Here's how the part is built. I have some questions about the finished solid (model axes, mm). A direction names the side the tool comes from. Round coordinates to 2 decimals unless told otherwise and drop trailing zeros. Write each loop counter-clockwise with the first axis right and the second up, starting at its lowest first coordinate (ties: lowest second). Pieces come first, ordered by that corner, then holes. Notation, with made-up numbers: (34, 23.5) - (48, 23.5) arc R25 ccw to (48, 41.5) - close; hole circle Ø2 at (29.25, 19). An arc over 180 degrees is marked (long way). Return JSON: item names as keys, results as strings. Group by question number.
```python
from build123d import *

# Parameters (mm, degrees)
SKETCH1_W           = 12.7
SKETCH1_H           = 12.7
BOSS_EXTRUDE1_DEPTH = 1.7
CHAMFER3_SIZE       = 1.41
SKETCH2_R           = 1.2
CUT_EXTRUDE2_DEPTH  = 2.7
SKETCH3_R           = 3.15
SKETCH3_R_2         = 2.2
BOSS_EXTRUDE2_DEPTH = 7.8
SKETCH4_R           = 0.64
BOSS_EXTRUDE3_DEPTH = 5


with BuildPart() as part:
    # Sketch1 → Boss-Extrude1 (new body)
    with BuildSketch(Plane(origin=(0, 0, 0), x_dir=(0, 1, 0), z_dir=(0, 0, 1))):
        Rectangle(SKETCH1_W, SKETCH1_H)
    extrude(amount=BOSS_EXTRUDE1_DEPTH)

    # Chamfer3
    chamfer3_edges = [part.edges().sort_by_distance(p)[0] for p in [
        (6.35, 6.35, 0.85),
        (6.35, -6.35, 0.85),
        (-6.35, -6.35, 0.85),
        (-6.35, 6.35, 0.85),
    ]]
    chamfer(chamfer3_edges, length=CHAMFER3_SIZE)

    # Sketch2 → Cut-Extrude2 (cut, through all)
    with BuildSketch(Plane.XY.offset(1.7)):
        with Locations((-4.35, 4.35)):
            Circle(SKETCH2_R)
        with Locations((-4.35, -4.35)):
            Circle(SKETCH2_R)
        with Locations((4.35, -4.35)):
            Circle(SKETCH2_R)
        with Locations((4.35, 4.35)):
            Circle(SKETCH2_R)
    extrude(amount=-CUT_EXTRUDE2_DEPTH, mode=Mode.SUBTRACT)

    # Sketch3 → Boss-Extrude2 (add)
    with BuildSketch(Plane.XY.offset(1.7)):
        Circle(SKETCH3_R)
        Circle(SKETCH3_R_2, mode=Mode.SUBTRACT)
    extrude(amount=BOSS_EXTRUDE2_DEPTH)

    # Sketch4 → Boss-Extrude3 (add)
    with BuildSketch(Plane(origin=(0, 0, 0), x_dir=(1, 0, 0), z_dir=(0, 0, -1))):
        Circle(SKETCH4_R)
    extrude(amount=BOSS_EXTRUDE3_DEPTH)


solid = part.part
```
1) Will these pins go through, and if not, where does the flat tip stop? pin 1 Ø3 at (x, y) = (4.35, -4.35) entering from -Z; pin 2 Ø4 at (x, y) = (-4.35, 4.35) entering from +Z; pin 3 Ø1 at (y, z) = (-2.5, 3.5) entering from +X.
2) Imagine slicing it at C-C (y = 0). Please give me the cut outline in (x, z).
3) Imagine slicing it at D-D (z = 5.75). Please give me the cut outline in (x, y).
4) For faces 1 (the cylindrical face through (-4.51, -3.16, 0.86)), 2 (the flat face through (0, 0, 1.7)), 3 (the cylindrical face through (-0.64, -0.03, -2.46)), which set-ups out of +Z, -Z, +X, -X, +Y, -Y let a thin tool reach every point of the face, with its end or its side?
5) I need wall thicknesses on line 1 along Y through (x, z) = (-4.35, 1.1); line 2 along Y through (x, z) = (0, 7.25); line 3 along Z through (x, y) = (1.25, 1.5). Which ranges of each line are inside material? Lowest first, please.
6) Imagine slicing it at A-A (x = 4.35). Please give me the cut outline in (y, z).
Results found:
{
 "1": {"pin 1": "stops at z = 0", "pin 2": "stops at z = 1.7", "pin 3": "stops at x = 2.43"},
 "2": {"outline": "(-6.35, 0) - (-0.64, 0) - (-0.64, -5) - (0.64, -5) - (0.64, 0) - (6.35, 0) - (6.35, 1.7) - (3.15, 1.7) - (3.15, 9.5) - (2.2, 9.5) - (2.2, 1.7) - (-2.2, 1.7) - (-2.2, 9.5) - (-3.15, 9.5) - (-3.15, 1.7) - (-6.35, 1.7) - close"},
 "3": {"outline": "circle Ø6.3 at (0, 0); hole circle Ø4.4 at (0, 0)"},
 "4": {"face 1": "+Z, -Z", "face 2": "+Z", "face 3": "-Z"},
 "5": {"line 1": "y = -6.35 to -5.55, -3.15 to 3.15, 5.55 to 6.35", "line 2": "y = -3.15 to -2.2, 2.2 to 3.15", "line 3": "z = 0 to 1.7"},
 "6": {"outline": "(-6.35, 0) - (-5.55, 0) - (-5.55, 1.7) - (-6.35, 1.7) - close; (-3.15, 0) - (3.15, 0) - (3.15, 1.7) - (-3.15, 1.7) - close; (5.55, 0) - (6.35, 0) - (6.35, 1.7) - (5.55, 1.7) - close"}
}
